from build123d import *

# Parameters (mm, degrees)
SKETCH_1_R          = 1.6
SKETCH_1_R_2        = 5.025
EXTRUDE_1_DEPTH     = 3
SKETCH_2_R          = 1.6
CUT_EXTRUDE_1_DEPTH = 124.535581919
FILLET_1_R          = 1
EXTRUDE_START       = -3
EXTRUDE_2_DEPTH     = 3
CHAMFER_1_SIZE      = 1.75


with BuildPart() as part:
    # ｽｹｯﾁ1 → ﾎﾞｽ - 押し出し1 (new body)
    with BuildSketch(Plane.XY):
        with BuildLine():
            Line((-2.227171492, 19.875605831), (86.459242762, 29.813408746))
            ThreePointArc((86.459242762, 29.813408746), (119.8, 0), (86.459242762, -29.813408746))
            Line((86.459242762, -29.813408746), (-2.227171492, -19.875605831))
            ThreePointArc((-2.227171492, -19.875605831), (-20, 0), (-2.227171492, 19.875605831))
        make_face()
        Circle(SKETCH_1_R, mode=Mode.SUBTRACT)
        with Locations((89.8, 0)):
            Circle(SKETCH_1_R_2, mode=Mode.SUBTRACT)
    extrude(amount=EXTRUDE_1_DEPTH)

    # ｽｹｯﾁ2 → ｶｯﾄ - 押し出し1 (cut, through all)
    with BuildSketch(Plane.XY.offset(3)):
        with Locations((21.127828075, 17.209804787)):
            Circle(SKETCH_2_R)
        with Locations((21.127828075, -17.209804787)):
            Circle(SKETCH_2_R)
        with Locations((60.046685431, -21.570877871)):
            Circle(SKETCH_2_R)
        with Locations((60.046685431, 21.570877871)):
            Circle(SKETCH_2_R)
        Polygon((24.311632117, -17.566567628), (56.056085363, -21.123709076), (38.398951009, -3.529263334), align=None)
        Polygon((24.311632117, 17.566567628), (56.056085363, 21.123709076), (38.398951009, 3.529263334), align=None)
        with BuildLine():
            Line((34.857112989, 0), (22.640031329, -12.173707016))
            ThreePointArc((22.640031329, -12.173707016), (21.34147622, -12.270762122), (21.047953505, -11.002097675))
            ThreePointArc((21.047953505, -11.002097675), (23.75, 0), (21.047953505, 11.002097675))
            ThreePointArc((21.047953505, 11.002097675), (21.34147622, 12.270762122), (22.640031329, 12.173707016))
            Line((22.640031329, 12.173707016), (34.857112989, 0))
        make_face()
        with BuildLine():
            Line((58.927113914, 16.926017866), (41.940789029, 0))
            Line((41.940789029, 0), (58.927113914, -16.926017866))
            ThreePointArc((58.927113914, -16.926017866), (60.230336409, -17.019617306), (60.513751544, -15.744146574))
            ThreePointArc((60.513751544, -15.744146574), (56.55, 0), (60.513751544, 15.744146574))
            ThreePointArc((60.513751544, 15.744146574), (60.230336409, 17.019617306), (58.927113914, 16.926017866))
        make_face()
    extrude(amount=-CUT_EXTRUDE_1_DEPTH, mode=Mode.SUBTRACT)

    # ﾌｨﾚｯﾄ1
    fillet_1_edges = [part.edges().sort_by_distance(p)[0] for p in [
        (41.940789029, 0, 1.5),
        (56.056085363, 21.123709076, 1.5),
        (38.398951009, 3.529263334, 1.5),
        (24.311632117, 17.566567628, 1.5),
        (34.857112989, 0, 1.5),
        (38.398951009, -3.529263334, 1.5),
        (56.056085363, -21.123709076, 1.5),
        (24.311632117, -17.566567628, 1.5),
    ]]
    fillet(fillet_1_edges, radius=FILLET_1_R)

    # ｽｹｯﾁ3 → ﾎﾞｽ - 押し出し2 (add)
    with BuildSketch(Plane.XY.offset(3).offset(EXTRUDE_START)):
        with BuildLine():
            Line((1.298294376, 21.801707083), (81.979371475, 30.430868694))
            ThreePointArc((81.979371475, 30.430868694), (91.382052123, 30.32494875), (100.500192923, 28.026877661))
            ThreePointArc((100.500192923, 28.026877661), (93.586587742, 29.760069779), (86.459242762, 29.813408746))
            Line((86.459242762, 29.813408746), (-2.227171492, 19.875605831))
            ThreePointArc((-2.227171492, 19.875605831), (-9.804357498, 17.431998567), (-15.827921381, 12.226074789))
            ThreePointArc((-15.827921381, 12.226074789), (-8.243504916, 18.764300705), (1.298294376, 21.801707083))
        make_face()
        with BuildLine():
            Line((1.298294376, -21.801707083), (81.979371475, -30.430868694))
            ThreePointArc((81.979371475, -30.430868694), (91.382052123, -30.32494875), (100.500192923, -28.026877661))
            ThreePointArc((100.500192923, -28.026877661), (93.586587742, -29.760069779), (86.459242762, -29.813408746))
            Line((86.459242762, -29.813408746), (-2.227171492, -19.875605831))
            ThreePointArc((-2.227171492, -19.875605831), (-9.804357498, -17.431998567), (-15.827921381, -12.226074789))
            ThreePointArc((-15.827921381, -12.226074789), (-8.243504916, -18.764300705), (1.298294376, -21.801707083))
        make_face()
    extrude(amount=EXTRUDE_2_DEPTH)

    # 面取り1
    chamfer_1_edges = [part.edges().sort_by_distance(p)[0] for p in [
        (-1.6, 0, 3),
        (19.527828075, 17.209804787, 3),
        (58.446685431, 21.570877871, 3),
        (58.446685431, -21.570877871, 3),
        (19.527828075, -17.209804787, 3),
    ]]
    chamfer(chamfer_1_edges, length=CHAMFER_1_SIZE)


solid = part.part
Geometry check sheet. Reference: the model listing, model coordinates, mm. A direction names the side the tool comes from. Coordinates: 2 decimals unless noted, no trailing zeros. Order: outer loops, then holes, each group sorted by start corner. A loop starts at its lowest first (then second) coordinate and runs counter-clockwise, first axis right, second up. Notation, with made-up numbers: (34, 11.25) -> (54, 11.25) arc R19 ccw to (54, 36.25) -> close; hole circle Ø9 at (73.5, 88.5). An arc over 180 degrees is marked (long way). Use a Markdown table: item, result. Add a question column.
1. Set-up check for faces 5 (the face through (56.55, -0.23, 1.52)), 6 (the face through (91.25, -30.34, 1.48)): record each of +Z, -Z, +X, -X, +Y, -Y from which the full face is reachable in a straight line by a thin tool's end or side.
2. Mould release check, pull along Y, two halves, no side actions. Record for faces 1 (the face through (58.45, 21.64, 0.63)), 2 (the face through (22.654, -16.729, 0.634)), 3 (the face through (66, 0, 0)), 4 (the face through (119.796, 0.507, 1.479)): pulls with the +Y half, pulls with the -Y half, needs draft (parallel to the pull), parting line crosses it, or undercut.
3. Cross-section at C-C (y = 8.5). Enter the section's corners in (x, z), and give its area (3 significant figures).
4. Cross-section at D-D (z = 2.4). Give the number of separate pieces and of enclosed holes in the cut face, and give its area (3 significant figures).
5. Material ranges on L1, parallel to X at y = 2.5, z = 2.05; L2, parallel to X at y = 8, z = 0.6; L3, parallel to Y at x = 32, z = 2.4, recorded low to high.
6. Cross-section at B-B (x = 47). Enter the section's corners in (y, z), and give its area (3 significant figures).
7. Cross-section at A-A (x = 0). Enter the section's corners in (y, z), and give its area (3 significant figures).
8. Go/stop test with flat-tipped pins: pin 1 Ø3.5 at (x, y) = (21.13, 17.21) entering from +Z; pin 2 Ø1 at (x, z) = (29, 2) entering from +Y; pin 3 Ø1.5 at (y, z) = (23.5, 1.5) entering from +X. Record where each tip stops, or that it passes through.
Filled sheet:
| question | item | result |
|---|---|---|
| 1 | face 5 | +Z, -Z |
| 1 | face 6 | +Z, -Z, -Y |
| 2 | face 1 | undercut |
| 2 | face 2 | undercut |
| 2 | face 3 | needs draft |
| 2 | face 4 | parting line crosses it |
| 3 | outline | (-18.1, 0) -> (22.18, 0) -> (22.18, 3) -> (-18.1, 3) -> close; (26.33, 0) -> (33.41, 0) -> (33.41, 3) -> (26.33, 3) -> close; (43.39, 0) -> (50.47, 0) -> (50.47, 3) -> (43.39, 3) -> close; (57.65, 0) -> (118.57, 0) -> (118.57, 3) -> (57.65, 3) -> close |
| 3 | area | 346 mm2 |
| 4 | separate pieces | 1 |
| 4 | enclosed holes | 10 |
| 4 | area | 5,720 mm2 |
| 5 | L1 | -19.84 to 23.62, 32.35 to 44.45, 56.64 to 85.44, 94.16 to 119.7 |
| 5 | L2 | -18.33 to 22.36, 26.83 to 33.91, 42.89 to 49.97, 57.53 to 118.71 |
| 5 | L3 | -25.09 to -18.43, -9.91 to -2.85, 2.85 to 9.91, 18.43 to 25.09 |
| 6 | outline | (-26.69, 0) -> (-20.11, 0) -> (-20.11, 3) -> (-26.69, 3) -> close; (-12.1, 0) -> (-5.04, 0) -> (-5.04, 3) -> (-12.1, 3) -> close; (5.04, 0) -> (12.1, 0) -> (12.1, 3) -> (5.04, 3) -> close; (20.11, 0) -> (26.69, 0) -> (26.69, 3) -> (20.11, 3) -> close |
| 6 | area | 81.8 mm2 |
| 7 | outline | (-21.63, 0) -> (-1.6, 0) -> (-1.6, 1.25) -> (-3.35, 3) -> (-21.63, 3) -> close; (1.6, 0) -> (21.63, 0) -> (21.63, 3) -> (3.35, 3) -> (1.6, 1.25) -> close |
| 7 | area | 117 mm2 |
| 8 | pin 1 | z = 1.4 |
| 8 | pin 2 | y = 24.82 |
| 8 | pin 3 | x = 109.36 |
